from build123d import *

# Parameters (mm, degrees)
F0_R     = 14.2875
F1_DEPTH = 31.75
F2_DEPTH = 4.7625
F4_DEPTH = 25.4
F5_DEPTH = 25.4
F6_DEPTH = 4.7752
F3_R     = 5.5626
F7_DEPTH = 25.4


with BuildPart() as f1:
    # F0 (on Front) → F1 (new body, symmetric)
    with BuildSketch(Plane.XZ):
        with BuildLine():
            Line((38.1, 28.575), (0, 28.575))
            ThreePointArc((0, 28.575), (-27.3235693319, -8.3638020041), (15.9950252975, -23.6788891364))
            ThreePointArc((15.9950252975, -23.6788891364), (25.7719232537, -12.3425522809), (28.4756083945, 2.38125))
            ThreePointArc((28.4756083945, 2.38125), (30.9572676717, 9.6234554837), (37.9674778593, 12.7))
            Line((37.9674778593, 12.7), (69.85, 12.7))
            Line((69.85, 12.7), (96.8502, 12.7))
            Line((96.8502, 12.7), (96.8502, 33.3502))
            Line((96.8502, 33.3502), (38.1, 33.3502))
            Line((38.1, 33.3502), (38.1, 28.575))
        make_face()
        Circle(F0_R, mode=Mode.SUBTRACT)
    extrude(amount=F1_DEPTH, both=True)

    # F0 (on Front) → F2 (join, symmetric)
    with BuildSketch(Plane.XZ):
        with BuildLine():
            ThreePointArc((28.4756083945, 2.38125), (25.7719232537, -12.3425522809), (15.9950252975, -23.6788891364))
            Line((15.9950252975, -23.6788891364), (69.85, 12.7))
            Line((69.85, 12.7), (37.9674778593, 12.7))
            ThreePointArc((37.9674778593, 12.7), (30.9572676717, 9.6234554837), (28.4756083945, 2.38125))
        make_face()
    extrude(amount=F2_DEPTH, both=True)

    # F3 (on face) → F4 (cut)
    with BuildSketch(Plane.XY.offset(33.3502)):
        with BuildLine():
            ThreePointArc((50.8, 31.75), (54.0586759125, 31.3248128824), (57.0991554441, 30.0777214642))
            Line((57.0991554441, 30.0777214642), (90.4493554441, 11.0277214642))
            ThreePointArc((90.4493554441, 11.0277214642), (95.1340352623, 6.3753715915), (96.8502, 0))
            Line((96.8502, 0), (96.8502, 31.75))
            Line((96.8502, 31.75), (50.8, 31.75))
        make_face()
    extrude(amount=-F4_DEPTH, mode=Mode.SUBTRACT)

    # F3 (on face) → F5 (cut)
    with BuildSketch(Plane.XY.offset(33.3502)):
        with BuildLine():
            Line((96.8502, -31.75), (96.8502, 0))
            ThreePointArc((96.8502, 0), (95.1340352623, -6.3753715915), (90.4493554441, -11.0277214642))
            Line((90.4493554441, -11.0277214642), (57.0991554441, -30.0777214642))
            ThreePointArc((57.0991554441, -30.0777214642), (54.0586759125, -31.3248128824), (50.8, -31.75))
            Line((50.8, -31.75), (96.8502, -31.75))
        make_face()
    extrude(amount=-F5_DEPTH, mode=Mode.SUBTRACT)

    # F3 (on face) → F6 (cut)
    with BuildSketch(Plane.XY.offset(33.3502)):
        with BuildLine():
            ThreePointArc((50.8, -31.75), (41.8197438789, -28.0302561211), (38.1, -19.05))
            Line((38.1, -19.05), (38.1, -31.75))
            Line((38.1, -31.75), (50.8, -31.75))
        make_face()
        with BuildLine():
            ThreePointArc((38.1, 19.05), (41.8197438789, 28.0302561211), (50.8, 31.75))
            Line((50.8, 31.75), (38.1, 31.75))
            Line((38.1, 31.75), (38.1, 19.05))
        make_face()
    extrude(amount=-F6_DEPTH, mode=Mode.SUBTRACT)

    # F3 (on face) → F7 (cut)
    with BuildSketch(Plane.XY.offset(33.3502)):
        with Locations((84.1502, 0)):
            Circle(F3_R)
        with Locations((50.8, 19.05)):
            Circle(F3_R)
        with Locations((50.8, -19.05)):
            Circle(F3_R)
    extrude(amount=-F7_DEPTH, mode=Mode.SUBTRACT)


solid = f1.part
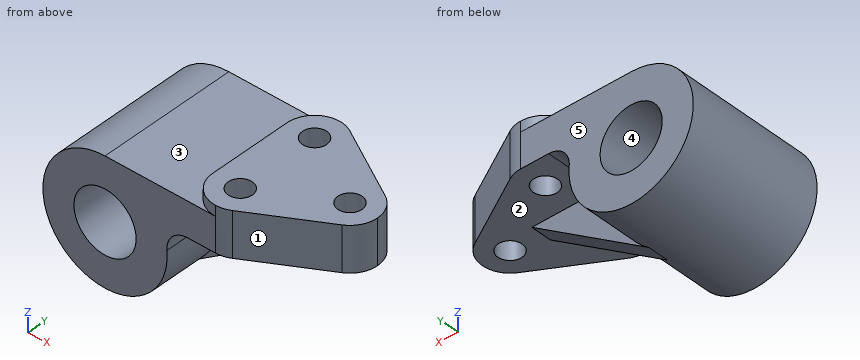
Work out the finished part from the listing and answer in its coordinate system (mm). Face numbers are marked on the shaded views. A direction names the side the tool comes from. Round coordinates to 2 decimals unless told otherwise and drop trailing zeros. Write each loop counter-clockwise with the first axis right and the second up, starting at its lowest first coordinate (ties: lowest second). Pieces come first, ordered by that corner, then holes.
1) Given pin 1 Ø8 at (x, y) = (83.5, -3.5) entering from -Z; pin 2 Ø1.4 at (y, z) = (0, 31) entering from -X; pin 3 Ø8 at (x, y) = (-6, 2.5) entering from -Z, each flat-ended and moving along its own axis, determine where each tip first touches the part or whether it passes through.
2) Straight lines are drawn through the part: line 1 (Y direction, x = 50.8, z = 23.25); line 2 (Z direction, x = 0, y = -11) (1 decimal); line 3 (Y direction, x = 54.5, z = 7). For each, find the intervals that lie inside material, in ascending order.
3) A cutting plane is placed at A-A (y = -16.5). Give the number of separate pieces and of enclosed holes in the cut face, plus the area to 3 significant figures.
4) The mould has two halves that part along Z. Classify the marked faces 3, 4 and 5: pulls with the +Z half, pulls with the -Z half, needs draft (parallel to the pull), parting line crosses it, or undercut.
5) A cutting plane is placed at D-D (x = 3). Give the vertices of the cut face in (y, z) (3 decimals).
6) A cutting plane is placed at C-C (z = 21). Give the vertices of the cut face in (x, y).
7) A tool of negligible diameter and unlimited length cuts with its end or side. For the marked faces 1 and 2, from which of +Z, -Z, +X, -X, +Y, -Y can it reach the whole face along a straight path? Write none if from no direction.
8) A cutting plane is placed at B-B (z = 9). Give the vertices of the cut face in (x, y).
Completed:
1. pin 1: stops at z = 12.7
1. pin 2: stops at x = 38.1
1. pin 3: stops at z = -28.5
2. line 1: y = -31.75 to -24.61, -13.49 to 13.49, 24.61 to 31.75
2. line 2: z = -28.6 to -14.3, 14.3 to 28.6
2. line 3: y = -4.76 to 4.76
3. separate pieces: 2
3. enclosed holes: 1
3. area: 2,950 mm2
4. face 3: pulls with the +Z half
4. face 4: undercut
4. face 5: needs draft
5. outline: (-31.75, -28.417) - (31.75, -28.417) - (31.75, -13.969) - (-31.75, -13.969) - close; (-31.75, 13.969) - (31.75, 13.969) - (31.75, 28.575) - (-31.75, 28.575) - close
6. outline: (-19.38, -31.75) - (50.8, -31.75) arc R12.7 ccw to (57.1, -30.08) - (90.45, -11.03) arc R12.7 ccw to (90.45, 11.03) - (57.1, 30.08) arc R12.7 ccw to (50.8, 31.75) - (-19.38, 31.75) - close; hole circle Ø11.13 at (50.8, -19.05); hole circle Ø11.13 at (50.8, 19.05); hole circle Ø11.13 at (84.15, 0)
7. face 1: +Z, -Z, +X, -Y
7. face 2: -Z, +X
8. outline: (-27.12, -31.75) - (-11.1, -31.75) - (-11.1, 31.75) - (-27.12, 31.75) - close; (11.1, -31.75) - (30.43, -31.75) - (30.43, -4.76) - (64.37, -4.76) - (64.37, 4.76) - (30.43, 4.76) - (30.43, 31.75) - (11.1, 31.75) - close
